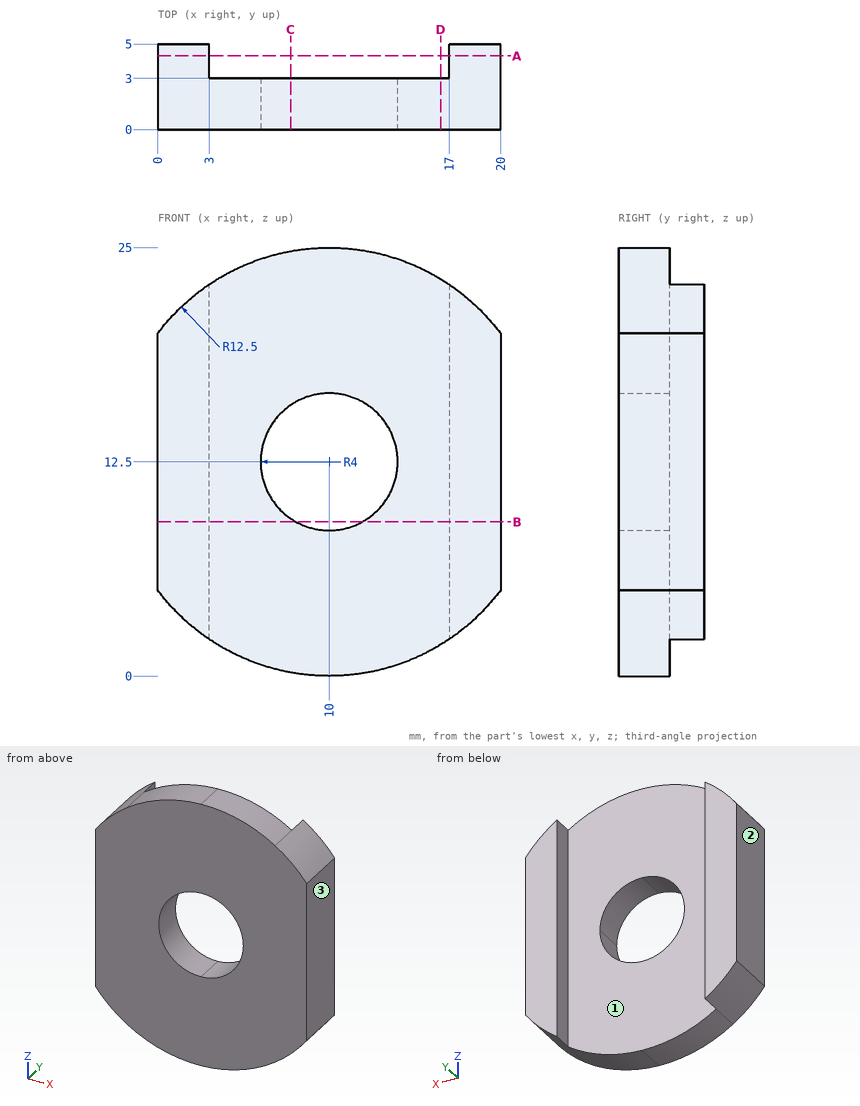
Source: three-view drawing plus pictorial views. Frame: mm from the lowest corner of the part. Round coordinates to 2 decimals unless told otherwise and drop trailing zeros. Order: outer loops, then holes, each group sorted by start corner. A loop starts at its lowest first (then second) coordinate and runs counter-clockwise, first axis right, second up. Notation, with made-up numbers: (-27, 42) - (-11, 42) arc R17 cw to (-11, 50) - close; hole circle Ø9 at (22, -36.5). An arc over 180 degrees is marked (long way). Answer in a Markdown table with one row per item.
Item 1: Mould query, pull axis X, two halves, no side actions, for the marked faces 1, 2 and 3. Classes: released by +X, released by -X, zero draft, split by the parting line, or undercut.
Model answer:
| item | result |
|---|---|
| face 1 | undercut |
| face 2 | released by -X |
| face 3 | released by +X |
Item 2: Pin query (flat end, axial travel): pin 1 (1.5 mm diameter, centred on x = 4, z = 7.5, fed in from +Y). Return the tip coordinate at first contact, or that it passes through.
Model answer:
| item | result |
|---|---|
| pin 1 | stops at y = 3 |
Item 3: Line query: line 1 (X direction, y = 4.35, z = 14.5); line 2 (Y direction, x = 6.75, z = 16.75); line 3 (Z direction, x = 8.25, y = 1.35). Output: solid intervals per line, ascending.
Model answer:
| item | result |
|---|---|
| line 1 | x = 0 to 3, 17 to 20 |
| line 2 | y = 0 to 3 |
| line 3 | z = 0.12 to 8.9, 16.1 to 24.88 |
Item 4: Section query C-C (x = 7.75). Return the cut outline in (y, z).
Model answer:
| item | result |
|---|---|
| outline | (0, 0.2) - (3, 0.2) - (3, 9.19) - (0, 9.19) - close; (0, 15.81) - (3, 15.81) - (3, 24.8) - (0, 24.8) - close |
Item 5: Section query A-A (y = 4.3). Return the cut outline in (x, z), then the cut area to 3 significant figures.
Model answer:
| item | result |
|---|---|
| outline | (0, 5) arc R12.5 ccw to (3, 2.14) - (3, 22.86) arc R12.5 ccw to (0, 20) - close; (17, 2.14) arc R12.5 ccw to (20, 5) - (20, 20) arc R12.5 ccw to (17, 22.86) - close |
| area | 109 mm² |
Item 6: Section query D-D (x = 16.5). Return the cut outline in (y, z), then the cut area to 3 significant figures.
Model answer:
| item | result |
|---|---|
| outline | (0, 1.82) - (3, 1.82) - (3, 23.18) - (0, 23.18) - close |
| area | 64.1 mm² |
Item 7: Section query B-B (z = 9). Return the cut outline in (x, y).
Model answer:
| item | result |
|---|---|
| outline | (0, 0) - (8.06, 0) - (8.06, 3) - (3, 3) - (3, 5) - (0, 5) - close; (11.94, 0) - (20, 0) - (20, 5) - (17, 5) - (17, 3) - (11.94, 3) - close |
